Input: part model. Units: mm. Frame: model coordinates. Face numbers are marked on the shaded views. A direction names the side the tool comes from. Coordinates: 2 decimals unless noted, no trailing zeros. Order: outer loops, then holes, each group sorted by start corner. A loop starts at its lowest first (then second) coordinate and runs counter-clockwise, first axis right, second up. Notation, with made-up numbers: (-32.75, -20) -> (18.25, -20) arc R14 ccw to (18.25, -12) -> close; hole circle Ø7 at (14, 77). An arc over 180 degrees is marked (long way). One line per item, written item: value. Start each with the question number.
from build123d import *

# Parameters (mm, degrees)
SKETCH2_W           = 18
SKETCH2_H           = 24
SKETCH2_R           = 1
BOSS_EXTRUDE2_DEPTH = 2.5
SKETCH4_W           = 24
SKETCH4_H           = 2.5
BOSS_EXTRUDE3_DEPTH = 2.5
SKETCH6_W           = 2.5
SKETCH6_H           = 24
BOSS_EXTRUDE5_DEPTH = 17
SKETCH7_W           = 24
SKETCH7_H           = 2.5
BOSS_EXTRUDE6_DEPTH = 18


with BuildPart() as part:
    # Sketch2 → Boss-Extrude2 (new body)
    with BuildSketch(Plane(origin=(0, 0, 0), x_dir=(1, 0, 0), z_dir=(0, 1, 0))):
        with Locations((-11, 4)):
            Rectangle(SKETCH2_W, SKETCH2_H)
        with Locations(Location((-17, -6, 0), (0, 0, 270))):
            Circle(SKETCH2_R, mode=Mode.SUBTRACT)
        with Locations(Location((-17, -2, 0), (0, 0, 270))):
            Circle(SKETCH2_R, mode=Mode.SUBTRACT)
        with Locations(Location((-17, 2, 0), (0, 0, 270))):
            Circle(SKETCH2_R, mode=Mode.SUBTRACT)
        with Locations(Location((-17, 6, 0), (0, 0, 270))):
            Circle(SKETCH2_R, mode=Mode.SUBTRACT)
        with Locations(Location((-17, 10, 0), (0, 0, 270))):
            Circle(SKETCH2_R, mode=Mode.SUBTRACT)
        with Locations(Location((-17, 14, 0), (0, 0, 270))):
            Circle(SKETCH2_R, mode=Mode.SUBTRACT)
        with Locations(Location((-13, -4, 0), (0, 0, 270))):
            Circle(SKETCH2_R, mode=Mode.SUBTRACT)
        with Locations(Location((-13, 0, 0), (0, 0, 270))):
            Circle(SKETCH2_R, mode=Mode.SUBTRACT)
        with Locations(Location((-13, 4, 0), (0, 0, 270))):
            Circle(SKETCH2_R, mode=Mode.SUBTRACT)
        with Locations(Location((-13, 8, 0), (0, 0, 270))):
            Circle(SKETCH2_R, mode=Mode.SUBTRACT)
        with Locations(Location((-13, 12, 0), (0, 0, 270))):
            Circle(SKETCH2_R, mode=Mode.SUBTRACT)
        with Locations(Location((-9, -6, 0), (0, 0, 270))):
            Circle(SKETCH2_R, mode=Mode.SUBTRACT)
        with Locations(Location((-9, -2, 0), (0, 0, 270))):
            Circle(SKETCH2_R, mode=Mode.SUBTRACT)
        with Locations(Location((-9, 2, 0), (0, 0, 270))):
            Circle(SKETCH2_R, mode=Mode.SUBTRACT)
        with Locations(Location((-9, 6, 0), (0, 0, 270))):
            Circle(SKETCH2_R, mode=Mode.SUBTRACT)
        with Locations(Location((-9, 10, 0), (0, 0, 270))):
            Circle(SKETCH2_R, mode=Mode.SUBTRACT)
        with Locations(Location((-9, 14, 0), (0, 0, 270))):
            Circle(SKETCH2_R, mode=Mode.SUBTRACT)
        with Locations(Location((-5, -4, 0), (0, 0, 270))):
            Circle(SKETCH2_R, mode=Mode.SUBTRACT)
        with Locations(Location((-5, 0, 0), (0, 0, 270))):
            Circle(SKETCH2_R, mode=Mode.SUBTRACT)
        with Locations(Location((-5, 4, 0), (0, 0, 270))):
            Circle(SKETCH2_R, mode=Mode.SUBTRACT)
        with Locations(Location((-5, 8, 0), (0, 0, 270))):
            Circle(SKETCH2_R, mode=Mode.SUBTRACT)
        with Locations(Location((-5, 12, 0), (0, 0, 270))):
            Circle(SKETCH2_R, mode=Mode.SUBTRACT)
    extrude(amount=BOSS_EXTRUDE2_DEPTH)

    # Sketch4 → Boss-Extrude3 (add)
    with BuildSketch(Plane.ZY.offset(20)):
        with Locations((-4, 1.25)):
            Rectangle(SKETCH4_W, SKETCH4_H)
    extrude(amount=BOSS_EXTRUDE3_DEPTH)

    # Sketch6 → Boss-Extrude5 (add)
    with BuildSketch(Plane.XZ):
        with Locations((-21.25, -4)):
            Rectangle(SKETCH6_W, SKETCH6_H)
    extrude(amount=BOSS_EXTRUDE5_DEPTH)

    # Sketch7 → Boss-Extrude6 (add)
    with BuildSketch(Plane(origin=(-20, 0, 0), x_dir=(0, 0, -1), z_dir=(1, 0, 0))):
        with Locations((4, -15.75)):
            Rectangle(SKETCH7_W, SKETCH7_H)
    extrude(amount=BOSS_EXTRUDE6_DEPTH)


solid = part.part
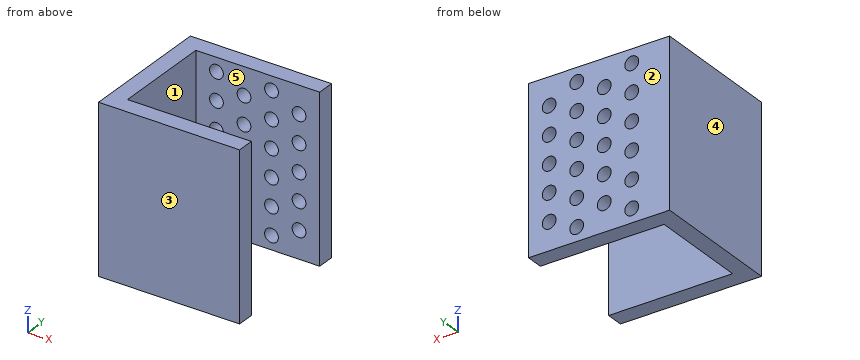
1) Ray query, line 1 along X through (y, z) = (1.8, -8); line 2 along X through (y, z) = (1.6, -14); line 3 along Y through (x, z) = (-9.5, -11.25). Return the intervals inside material, ascending. Write a range as from..to.
2) Section query C-C, the plane x = -5. Return the cut outline in (y, z), plus the area to 3 significant figures.
3) Mould query, pull axis Y, two halves, no side actions, for the marked faces 1, 2 and 3. Classes: +Y half, -Y half, draft (parallel to the pull), parting line (faces both ways), or undercut.
4) Section query D-D, the plane x = -9. State how many separate pieces and enclosed holes the cut face has, plus the area to 3 significant figures.
5) Access query for the marked faces 4 and 5. Directions: +Z, -Z, +X, -X, +Y, -Y. A direction counts if a zero-diameter tool reaches every point of the face in a straight line with its end or side. Return the directions, or none.
6) Pin query (flat end, axial travel): pin 1 Ø11.5 at (y, z) = (-8.5, -4) entering from +X; pin 2 Ø1.2 at (x, z) = (-13, 4) entering from +Y; pin 3 Ø8 at (y, z) = (-13, -9.5) entering from +X. Return the tip coordinate at first contact, or that it passes through.
7) Section query B-B, the plane z = -12. Return the cut outline in (x, y).
8) Section query A-A, the plane x = -19.5. Return the cut outline in (y, z), plus the area to 3 significant figures.
Entries:
1. line 1: x = -22.5..-14, -12..-6, -4..-2
1. line 2: x = -22.5..-18, -16..-10, -8..-2
1. line 3: y = -17..-14.5, 0..2.5
2. outline: (-17, -16) -> (-14.5, -16) -> (-14.5, 8) -> (-17, 8) -> close; (0, -16) -> (2.5, -16) -> (2.5, -13) -> (0, -13) -> close; (0, -11) -> (2.5, -11) -> (2.5, -9) -> (0, -9) -> close; (0, -7) -> (2.5, -7) -> (2.5, -5) -> (0, -5) -> close; (0, -3) -> (2.5, -3) -> (2.5, -1) -> (0, -1) -> close; (0, 1) -> (2.5, 1) -> (2.5, 3) -> (0, 3) -> close; (0, 5) -> (2.5, 5) -> (2.5, 8) -> (0, 8) -> close
2. area: 95.0 mm2
3. face 1: undercut
3. face 2: +Y half
3. face 3: -Y half
4. separate pieces: 8
4. enclosed holes: 0
4. area: 90.0 mm2
5. face 4: +Z, -Z, -X, +Y, -Y
5. face 5: +Z, -Z, +X
6. pin 1: stops at x = -20
6. pin 2: stops at y = -14.5
6. pin 3: stops at x = -2
7. outline: (-22.5, -17) -> (-2, -17) -> (-2, -14.5) -> (-20, -14.5) -> (-20, 0) -> (-14, 0) -> (-14, 2.5) -> (-22.5, 2.5) -> close; (-12, 0) -> (-6, 0) -> (-6, 2.5) -> (-12, 2.5) -> close; (-4, 0) -> (-2, 0) -> (-2, 2.5) -> (-4, 2.5) -> close
8. outline: (-17, -16) -> (-14.5, -16) -> (-14.5, 8) -> (-17, 8) -> close; (0, -16) -> (2.5, -16) -> (2.5, 8) -> (0, 8) -> close
8. area: 120 mm2
